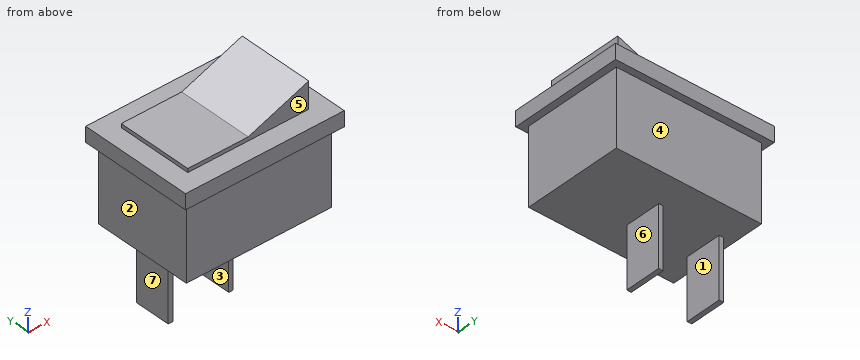
from build123d import *

# Parameters (mm, degrees)
SKETCH079_W  = 21
SKETCH079_H  = 15
PAD044_DEPTH = 2
SKETCH080_W  = 19.2
SKETCH080_H  = 13.2
PAD045_DEPTH = 10
SKETCH081_W  = 0.6
SKETCH081_H  = 4.8
PAD046_DEPTH = 8
PAD047_DEPTH = 5


with BuildPart() as part:
    # Sketch079 → Pad044 (new body)
    with BuildSketch(Plane.XY):
        Rectangle(SKETCH079_W, SKETCH079_H)
    extrude(amount=PAD044_DEPTH)

    # Sketch080 → Pad045 (join)
    with BuildSketch(Plane.XY):
        Rectangle(SKETCH080_W, SKETCH080_H)
    extrude(amount=-PAD045_DEPTH)

    # Sketch081 → Pad046 (join)
    with BuildSketch(Plane.XY.offset(-10)):
        Rectangle(SKETCH081_W, SKETCH081_H)
        with Locations((-8, 0)):
            Rectangle(SKETCH081_W, SKETCH081_H)
    extrude(amount=-PAD046_DEPTH)

    # Sketch082 → Pad047 (join, symmetric)
    with BuildSketch(Plane(origin=(0, 0, 2.5), x_dir=(1, 0, 0), z_dir=(0, -1, 0))):
        Polygon((-8, 0), (0, 0), (8, 3), (8, -1), (-8, -1), align=None)
    extrude(amount=PAD047_DEPTH, both=True)


solid = part.part
Can you work these out from the model? Positions are in its coordinate system, mm. Face numbers are marked on the shaded views. A direction names the side the tool comes from. Round coordinates to 2 decimals unless told otherwise and drop trailing zeros. Write each loop counter-clockwise with the first axis right and the second up, starting at its lowest first coordinate (ties: lowest second). Pieces come first, ordered by that corner, then holes. Notation, with made-up numbers: (36.5, 1.25) - (75.5, 1.25) arc R12 ccw to (75.5, 16.25) - close; hole circle Ø5 at (31, 29.5). An arc over 180 degrees is marked (long way). Write each question's results on one line, items separated by ' | '. Start each with the question number.
1) For pin 1 Ø8 at (x, z) = (-0.5, -0.5) entering from +Y; pin 2 Ø5.5 at (y, z) = (0, -13.5) entering from +X; pin 3 Ø0.5 at (x, z) = (-8, -16) entering from -Y; pin 4 Ø8 at (x, z) = (-4.5, -12) entering from -Y, each with a flat end and sliding along its axis, tell me the tip position at first contact or that it passes through.
2) Please list where these lines run through material, in increasing order: line 1 (X direction, y = -0.75, z = -14.5); line 2 (Z direction, x = -3, y = 0); line 3 (Y direction, x = -1.5, z = -0.75).
3) Suppose I cut it at C-C (y = -0.5). List the corners of the cut face in (x, z) for me, and give its area (3 significant figures).
4) Suppose I cut it at D-D (z = -9.25). List the corners of the cut face in (x, y) for me, and give its area (3 significant figures).
5) We'd pull the mould along X, two halves only. Please class the marked faces 1, 2, 3 and 4: released by +X, released by -X, zero draft, split by the parting line, or undercut.
6) Suppose I cut it at A-A (z = -11.75). List the corners of the cut face in (x, y) for me, and give its area (3 significant figures).
7) Which directions (+Z, -Z, +X, -X, +Y, -Y) give clear straight access to the entire face, cutting with the end or side of a thin tool? Please do the marked faces 5, 6 and 7.
8) Suppose I cut it at B-B (x = -8.75). List the corners of the cut face in (y, z) for me.
Here are the results:
1) pin 1: stops at y = 7.5 | pin 2: stops at x = 0.3 | pin 3: stops at y = -2.4 | pin 4: stops at y = -6.6
2) line 1: x = -8.3 to -7.7, -0.3 to 0.3 | line 2: z = -10 to 2.5 | line 3: y = -6.6 to 6.6
3) outline: (-10.5, 0) - (-9.6, 0) - (-9.6, -10) - (-8.3, -10) - (-8.3, -18) - (-7.7, -18) - (-7.7, -10) - (-0.3, -10) - (-0.3, -18) - (0.3, -18) - (0.3, -10) - (9.6, -10) - (9.6, 0) - (10.5, 0) - (10.5, 2) - (8, 2) - (8, 5.5) - (0, 2.5) - (-8, 2.5) - (-8, 2) - (-10.5, 2) - close | area: 264 mm2
4) outline: (-9.6, -6.6) - (9.6, -6.6) - (9.6, 6.6) - (-9.6, 6.6) - close | area: 253 mm2
5) face 1: undercut | face 2: released by -X | face 3: undercut | face 4: zero draft
6) outline: (-8.3, -2.4) - (-7.7, -2.4) - (-7.7, 2.4) - (-8.3, 2.4) - close; (-0.3, -2.4) - (0.3, -2.4) - (0.3, 2.4) - (-0.3, 2.4) - close | area: 5.76 mm2
7) face 5: +Z, +X, -X, -Y | face 6: -Z, +X, +Y, -Y | face 7: -Z, -X, +Y, -Y
8) outline: (-7.5, 0) - (-6.6, 0) - (-6.6, -10) - (6.6, -10) - (6.6, 0) - (7.5, 0) - (7.5, 2) - (-7.5, 2) - close
